Read the model definition and answer for the solid it produces. Units are mm, in the model's axes. A direction names the side the tool comes from. Coordinates: 2 decimals unless noted, no trailing zeros. Write each loop counter-clockwise with the first axis right and the second up, starting at its lowest first coordinate (ties: lowest second). Pieces come first, ordered by that corner, then holes.
from build123d import *

# Parameters (mm, degrees)
F1_DEPTH = 100


with BuildPart() as f1:
    # F0 (on Right) → F1 (new body)
    with BuildSketch(Plane.YZ):
        with BuildLine():
            Line((-5.472958, 37.051259), (-34.390154, 0))
            ThreePointArc((-34.390154, 0), (-41.9504, -2.979086), (-48.217188, 2.193884))
            Line((-48.217188, 2.193884), (-50.097297, 1.511836))
            ThreePointArc((-50.097297, 1.511836), (-42.263812, -4.954377), (-32.813505, -1.230519))
            Line((-32.813505, -1.230519), (-3.896309, 35.82074))
            ThreePointArc((-3.896309, 35.82074), (-0.46602, 37.3501), (2.720071, 35.361468))
            Line((2.720071, 35.361468), (23.738619, -1.000883))
            Line((23.738619, -1.000883), (25.47016, 0))
            Line((25.47016, 0), (4.451611, 36.362352))
            ThreePointArc((4.451611, 36.362352), (-0.327524, 39.345299), (-5.472958, 37.051259))
        make_face()
    extrude(amount=-F1_DEPTH)


solid = f1.part
Item 1: The part is cut by section C-C (y = -36). Give the vertices of the cut face in (x, z).
Item 2: For faces 4 (the flat face through (-49.3, 15.108, 17.927)), 5 (the flat face through (-49.3, -18.557, 17.036)), determine the directions among +Z, -Z, +X, -X, +Y, -Y from which every point of the face is accessible in a straight line to the end or side of a thin tool.
Item 3: Find the intervals of material crossed by probe 1 along Y at (x, z) = (-29, 0); probe 2 along Y at (x, z) = (-87, 5); probe 3 along Y at (x, z) = (-21, 34.5), in increasing order.
Item 4: Given pin 1 (12 mm diameter, centred on x = -64, y = 18, fed in from +Z); pin 2 (6 mm diameter, centred on x = -70.5, y = -13.5, fed in from +Z); pin 3 (5 mm diameter, centred on x = -14, y = -41.5, fed in from +Z); pin 4 (2 mm diameter, centred on y = -13.5, z = 20.5, fed in from -X), each flat-ended and moving along its own axis, determine where each tip first touches the part or whether it passes through.
Item 5: The part is cut by section B-B (z = 17). Give the vertices of the cut face in (x, y), and give its area (3 significant figures).
Item 6: Determine the mould class of faces 1 (the flat face through (-49.3, -19.729, 18.785)), 2 (the flat face through (-100, -15, 22)), 3 (the flat face through (0, -15, 22)) for opening direction X: +X half, -X half, draft (parallel to the pull), parting line (faces both ways), or undercut.
Item 7: The part is cut by section D-D (y = -23). Give the vertices of the cut face in (x, z).
Item 8: The part is cut by section A-A (x = -57.5). Give the vertices of the cut face in (y, z), and give its area (3 significant figures).
Answer:
1. outline: (-100, -3.91) - (0, -3.91) - (0, -1.55) - (-100, -1.55) - close
2. face 4: +Z, +X, -X, +Y
2. face 5: -Z, +X, -X
3. probe 1: y = -49.4 to -47, -34.39 to -31.85, 23.16 to 25.47
3. probe 2: y = -30.49 to -27.95, 20.27 to 22.58
3. probe 3: y = -7.46 to -4.93, 3.22 to 5.53
4. pin 1: stops at z = 23.3
4. pin 2: stops at z = 30.61
4. pin 3: stops at z = -2.36
4. pin 4: passes through
5. outline: (-100, -21.12) - (0, -21.12) - (0, -18.59) - (-100, -18.59) - close; (-100, 13.33) - (0, 13.33) - (0, 15.64) - (-100, 15.64) - close
5. area: 485 mm2
6. face 1: draft
6. face 2: -X half
6. face 3: +X half
7. outline: (-100, 11.34) - (0, 11.34) - (0, 14.59) - (-100, 14.59) - close
8. outline: (-50.1, 1.51) arc R10 ccw to (-32.81, -1.23) - (-3.9, 35.82) arc R4 cw to (2.72, 35.36) - (23.74, -1) - (25.47, 0) - (4.45, 36.36) arc R6 ccw to (-5.47, 37.05) - (-34.39, 0) arc R8 cw to (-48.22, 2.19) - close
8. area: 236 mm2
